Here's how the part is built. I have some questions about the finished solid (model axes, mm). Coordinates: 2 decimals unless noted, no trailing zeros. Order: outer loops, then holes, each group sorted by start corner. A loop starts at its lowest first (then second) coordinate and runs counter-clockwise, first axis right, second up. Notation, with made-up numbers: (-20, 52) - (-3, 52) arc R19 ccw to (-3, 59) - close; hole circle Ø10 at (28, 82.5). An arc over 180 degrees is marked (long way). Answer in a Markdown table with one row per item. Add a question column.
Item 1: Thinking about a two-plate mould opening in Y: for faces 1 (the cylindrical face through (-56.82, 119.46, 1.52)), 2 (the cylindrical face through (23.08, 105.26, 1.52)), 3 (the flat face through (24, 9, 0)), which applies, +Y half, -Y half, draft (parallel to the pull), parting line (faces both ways), or undercut?
Item 2: I want a section at A-A (y = 31). Please give me the cut outline in (x, z), plus the area to 3 significant figures.
Item 3: I want a section at C-C (z = 0.5). Count the separate pieces of the cut face and the enclosed holes in it, plus the area to 3 significant figures.
Item 4: If I drill on line 1 along X through (y, z) = (53.5, 1.5); line 2 along X through (y, z) = (96.5, 0.3); line 3 along Y through (x, z) = (78.5, 1.2), over which ranges is the centre line in solid material (lowest first)? Write a range as from..to.
Item 5: I want a section at B-B (x = -5). Please give me the cut outline in (y, z).
```python
from build123d import *

# Parameters (mm, degrees)
F0_W     = 249
F0_H     = 271
F0_W_2   = 227
F0_H_2   = 249
F1_DEPTH = 3
F2_W     = 97.5
F2_H     = 40
F2_R     = 11
F2_R_2   = 1.75
F2_W_2   = 3
F2_H_2   = 20
F2_W_3   = 13
F2_W_4   = 25
F2_H_3   = 3
F2_R_3   = 5
F2_W_5   = 7.7
F2_H_4   = 2.5
F3_DEPTH = 25
F4_W     = 249
F4_H     = 271
F5_DEPTH = 3


with BuildPart() as f1:
    # F0 (on Top) → F1 (new body)
    with BuildSketch(Plane.XY):
        Rectangle(F0_W, F0_H)
        Rectangle(F0_W_2, F0_H_2, mode=Mode.SUBTRACT)
        Rectangle(F0_W_2, F0_H_2)
    extrude(amount=F1_DEPTH)

    # F2 (on face) → F3 (cut)
    with BuildSketch(Plane.XY.offset(3)):
        with Locations((6.014311, 40.348687)):
            Rectangle(F2_W, F2_H)
        with Locations((-34.873512, 95.984109)):
            Circle(F2_R)
        with Locations((17.168977, 95.984109)):
            Circle(F2_R)
        with Locations((-40.735689, 67.848687)):
            Circle(F2_R_2)
        with Locations((52.764311, 67.848687)):
            Circle(F2_R_2)
        with Locations((52.764311, 12.848687)):
            Circle(F2_R_2)
        with Locations((-40.735689, 12.848687)):
            Circle(F2_R_2)
        with Locations((45.454934, -22.752056)):
            Rectangle(F2_W_2, F2_H_2)
        with Locations((84.206969, 95.984109)):
            Rectangle(F2_W_3, F2_H_2)
        with Locations((83.148815, -3.833046)):
            Rectangle(F2_W_4, F2_H_3)
        with Locations((84.014516, 52.88054)):
            Circle(F2_R_3)
        with Locations((84.000645, 25.185113)):
            Rectangle(F2_W_5, F2_H_4)
    extrude(amount=-F3_DEPTH, mode=Mode.SUBTRACT)

    # F4 (on face) → F5 (cut, through all)
    with BuildSketch(Plane.XY.offset(3)):
        Rectangle(F4_W, F4_H)
        with BuildLine():
            ThreePointArc((-61.096646, 108.972366), (-56.703248, 119.578968), (-46.096646, 123.972366))
            Line((-46.096646, 123.972366), (95.905387, 123.972366))
            ThreePointArc((95.905387, 123.972366), (106.511988, 119.578968), (110.905387, 108.972366))
            Line((110.905387, 108.972366), (110.905387, -50.685034))
            ThreePointArc((110.905387, -50.685034), (106.511988, -61.291636), (95.905387, -65.685034))
            Line((95.905387, -65.685034), (-46.096646, -65.685034))
            ThreePointArc((-46.096646, -65.685034), (-56.703248, -61.291636), (-61.096646, -50.685034))
            Line((-61.096646, -50.685034), (-61.096646, 108.972366))
        make_face(mode=Mode.SUBTRACT)
    extrude(amount=-F5_DEPTH, mode=Mode.SUBTRACT)


solid = f1.part
```
Values follow:
| question | item | result |
|---|---|---|
| 1 | face 1 | +Y half |
| 1 | face 2 | undercut |
| 1 | face 3 | draft |
| 2 | outline | (-61.1, 0) - (-42.74, 0) - (-42.74, 3) - (-61.1, 3) - close; (54.76, 0) - (110.91, 0) - (110.91, 3) - (54.76, 3) - close |
| 2 | area | 224 mm^2 |
| 3 | separate pieces | 1 |
| 3 | enclosed holes | 12 |
| 3 | area | 27,200 mm^2 |
| 4 | line 1 | x = -61.1..-42.74, 54.76..79.05, 88.98..110.91 |
| 4 | line 2 | x = -61.1..-45.86, -23.89..6.18, 28.16..77.71, 90.71..110.91 |
| 4 | line 3 | y = -65.69..-5.33, -2.33..85.98, 105.98..123.97 |
| 5 | outline | (-65.69, 0) - (20.35, 0) - (20.35, 3) - (-65.69, 3) - close; (60.35, 0) - (123.97, 0) - (123.97, 3) - (60.35, 3) - close |
